Check sheet for the modelled part. Datum: model origin and axes. Units: mm. Face numbers are marked on the shaded views. A direction names the side the tool comes from. Round coordinates to 2 decimals unless told otherwise and drop trailing zeros. Loops run counter-clockwise (first coordinate to the right, second up) from the corner with the lowest first, then second, coordinate; pieces in that order, holes last. Notation, with made-up numbers: (74.25, -30.75) -> (92.25, -30.75) arc R12 ccw to (92.25, -26.75) -> close; hole circle Ø2 at (-13, 23.5). An arc over 180 degrees is marked (long way). Use one line per item in the form item = value. Start each with the question number.
(1) Draft check along Z on the marked faces 1, 2 and 3. Enter one of: released by +Z, released by -Z, zero draft, split by the parting line, or undercut.
(2) Sectioned sample at C-C (y = -15.5). Record the cut outline in (x, z), and give its area (3 significant figures).
(3) Go/stop test with flat-tipped pins: pin 1 (3 mm diameter, centred on x = -6.5, y = 21, fed in from -Z); pin 2 (0.9 mm diameter, centred on x = 9, z = -77.5, fed in from +Y); pin 3 (4 mm diameter, centred on x = 28, y = 9.5, fed in from -Z); pin 4 (0.9 mm diameter, centred on x = -1, z = -77.5, fed in from -Y). Record where each tip stops, or that it passes through.
(4) Set-up check for the marked faces 4 and 5: record each of +Z, -Z, +X, -X, +Y, -Y from which the full face is reachable in a straight line by a thin tool's end or side.
(5) Sectioned sample at B-B (y = 16). Record the cut outline in (x, z).
(6) Sectioned sample at D-D (x = -3). Record the cut outline in (y, z), and give its area (3 significant figures).
(7) Sectioned sample at A-A (z = -43). Record the cut outline in (x, y), and give its area (3 significant figures).
(8) Material ranges on probe 1 along X at (y, z) = (27.8, -43); probe 2 along X at (y, z) = (26, 0); probe 3 along X at (y, z) = (16, -75), recorded low to high. Write a range as [from, to].
from build123d import *

# Parameters (mm, degrees)
SKETCH_1_R               = 5
EXTRUDE_1_DEPTH          = 30
EXTRUDE_1_2_DEPTH        = 30
EXTRUDE_1_3_DEPTH        = 30
EXTRUDE_1_4_DEPTH        = 30
EXTRUDE_START            = 18
SKETCH_2_R               = 5
EXTRUDE_2_DEPTH          = 18
SKETCH_3_R               = 2.1
CUT_EXTRUDE_1_DEPTH      = 5
EXTRUDE_START_2          = 20
EXTRUDE_3_DEPTH          = 10
EXTRUDE_3_2_DEPTH        = 10
CUT_EXTRUDE_2_DEPTH      = 102.257098517
CUT_EXTRUDE_2_DEPTH_BACK = 102.257098517
EXTRUDE_START_3          = -3
EXTRUDE_4_DEPTH          = 3
SKETCH_7_R               = 2.1
CUT_EXTRUDE_3_DEPTH      = 5
SKETCH_8_R               = 1.9
EXTRUDE_5_DEPTH          = 4
SKETCH_9_R               = 1.9
EXTRUDE_6_DEPTH          = 4
CHAMFER_1_SIZE           = 1


with BuildPart() as part:
    # Sketch 1 → Extrude 1 (new body)
    with BuildSketch(Plane(origin=(0, 0, 0), x_dir=(1, 0, 0), z_dir=(0, 1, 0))):
        with Locations(Location((30, 0, 0), (0, 0, 270))):
            Circle(SKETCH_1_R)
    extrude(amount=EXTRUDE_1_DEPTH)



with BuildPart() as body_2:
    # Sketch 1 → Extrude 1 2 (new body)
    with BuildSketch(Plane(origin=(0, 0, 0), x_dir=(1, 0, 0), z_dir=(0, 1, 0))):
        with Locations(Location((25, 77, 0), (0, 0, 270))):
            Circle(SKETCH_1_R)
    extrude(amount=EXTRUDE_1_2_DEPTH)


with BuildPart() as body_3:
    # Sketch 1 → Extrude 1 3 (new body)
    with BuildSketch(Plane(origin=(0, 0, 0), x_dir=(1, 0, 0), z_dir=(0, 1, 0))):
        with Locations(Location((-30, 0, 0), (0, 0, 90))):
            Circle(SKETCH_1_R)
    extrude(amount=EXTRUDE_1_3_DEPTH)


with BuildPart() as body_4:
    # Sketch 1 → Extrude 1 4 (new body)
    with BuildSketch(Plane(origin=(0, 0, 0), x_dir=(1, 0, 0), z_dir=(0, 1, 0))):
        with Locations(Location((-25, 77, 0), (0, 0, 90))):
            Circle(SKETCH_1_R)
    extrude(amount=EXTRUDE_1_4_DEPTH)


with BuildPart() as part_1:
    add(part.part)

    add(body_3.part)  # Extrude 2 merges body 3
    # Sketch 2 → Extrude 2 (add)
    with BuildSketch(Plane.XZ.offset(EXTRUDE_START)):
        with Locations(Location((-30, 0, 0), (0, 0, 270))):
            Circle(SKETCH_2_R)
        with Locations(Location((30, 0, 0), (0, 0, 270))):
            Circle(SKETCH_2_R)
    extrude(amount=-EXTRUDE_2_DEPTH)

    # Sketch 5 → Cut-Extrude 2 (cut, two sides: drawn at the far end of the back side and taken through both)
    with BuildSketch(Plane(origin=(0, 30, 0), x_dir=(1, 0, 0), z_dir=(0, 1, 0)).offset(-CUT_EXTRUDE_2_DEPTH_BACK)):
        with BuildLine():
            Line((-32.175491387, 4.50191484), (-25.273954776, 1.632328565))
            ThreePointArc((-25.273954776, 1.632328565), (-28.080374368, 4.61682114), (-32.175491387, 4.50191484))
        make_face()
        with BuildLine():
            Line((25.273954776, 1.632328565), (32.175491387, 4.50191484))
            ThreePointArc((32.175491387, 4.50191484), (28.080374368, 4.61682114), (25.273954776, 1.632328565))
        make_face()
    extrude(amount=CUT_EXTRUDE_2_DEPTH + CUT_EXTRUDE_2_DEPTH_BACK, mode=Mode.SUBTRACT)



with BuildPart() as cut_extrude_1_tool:
    # Sketch 3 → Cut-Extrude 1 (new body)
    with BuildSketch(Plane(origin=(0, 30, 0), x_dir=(1, 0, 0), z_dir=(0, 1, 0))):
        with Locations(Location((-25, 77, 0), (0, 0, 270))):
            Circle(SKETCH_3_R)
        with Locations(Location((25, 77, 0), (0, 0, 270))):
            Circle(SKETCH_3_R)
    extrude(amount=-CUT_EXTRUDE_1_DEPTH)


with BuildPart() as body_2_1:
    add(body_2.part)

    # Cut-Extrude 1: cut by cut_extrude_1_tool
    add(cut_extrude_1_tool.part, mode=Mode.SUBTRACT)


with BuildPart() as body_4_1:
    add(body_4.part)

    # Cut-Extrude 1: cut by cut_extrude_1_tool
    add(cut_extrude_1_tool.part, mode=Mode.SUBTRACT)


with BuildPart() as body_4_2:
    # Sketch 4 → Extrude 3 (new body)
    with BuildSketch(Plane(origin=(0, 0, 0), x_dir=(1, 0, 0), z_dir=(0, 1, 0)).offset(EXTRUDE_START_2)):
        with BuildLine():
            Line((23, 48), (28.159807037, 48))
            ThreePointArc((28.159807037, 48), (33.159807037, 43), (28.159807037, 38))
            Line((28.159807037, 38), (23, 38))
            Line((23, 38), (23, 48))
        make_face()
    extrude(amount=EXTRUDE_3_DEPTH)


with BuildPart() as body_5:
    # Sketch 4 → Extrude 3 2 (new body)
    with BuildSketch(Plane(origin=(0, 0, 0), x_dir=(1, 0, 0), z_dir=(0, 1, 0)).offset(EXTRUDE_START_2)):
        with BuildLine():
            Line((-23, 48), (-28.159807037, 48))
            ThreePointArc((-28.159807037, 48), (-33.159807037, 43), (-28.159807037, 38))
            Line((-28.159807037, 38), (-23, 38))
            Line((-23, 38), (-23, 48))
        make_face()
    extrude(amount=EXTRUDE_3_2_DEPTH)


with BuildPart() as part_2:
    add(part_1.part)

    add(body_2_1.part)  # Extrude 4 merges body 2

    add(body_4_1.part)  # Extrude 4 merges body 4

    add(body_4_2.part)  # Extrude 4 merges body 4 2

    add(body_5.part)  # Extrude 4 merges body 5
    # Sketch 6 → Extrude 4 (add)
    with BuildSketch(Plane(origin=(0, 30, 0), x_dir=(1, 0, 0), z_dir=(0, 1, 0)).offset(EXTRUDE_START_3)):
        Polygon((-29.42411231, 1.385046342), (-38.5, 5.158704907), (-38.5, 28.603878074), (-26.710319101, 42.386930811), (-23.632939423, 75.5), (23.632939423, 75.5), (26.710319101, 42.386930811), (38.5, 28.603878074), (38.5, 5.158704907), (29.42411231, 1.385046342), (30.57588769, -1.385046342), (41.5, 3.157084566), (41.5, 29.7119114), (29.609294973, 43.613069189), (26.367060577, 78.5), (-26.367060577, 78.5), (-29.609294973, 43.613069189), (-41.5, 29.7119114), (-41.5, 3.157084566), (-30.57588769, -1.385046342), align=None)
    extrude(amount=-EXTRUDE_4_DEPTH)

    # Sketch 7 → Cut-Extrude 3 (cut)
    with BuildSketch(Plane(origin=(0, 30, 0), x_dir=(1, 0, 0), z_dir=(0, 1, 0))):
        with Locations(Location((30, 0, 0), (0, 0, 270))):
            Circle(SKETCH_7_R)
        with Locations(Location((-30, 0, 0), (0, 0, 270))):
            Circle(SKETCH_7_R)
        with Locations(Location((28.159807037, 43, 0), (0, 0, 270))):
            Circle(SKETCH_7_R)
        with Locations(Location((-28.159807037, 43, 0), (0, 0, 270))):
            Circle(SKETCH_7_R)
        with Locations(Location((25, 77, 0), (0, 0, 270))):
            Circle(SKETCH_7_R)
        with Locations(Location((-25, 77, 0), (0, 0, 270))):
            Circle(SKETCH_7_R)
    extrude(amount=-CUT_EXTRUDE_3_DEPTH, mode=Mode.SUBTRACT)

    # Sketch 8 → Extrude 5 (add)
    with BuildSketch(Plane.XZ.offset(18)):
        with Locations(Location((-30, 0, 0), (0, 0, 270))):
            Circle(SKETCH_8_R)
        with Locations(Location((30, 0, 0), (0, 0, 270))):
            Circle(SKETCH_8_R)
    extrude(amount=EXTRUDE_5_DEPTH)

    # Sketch 9 → Extrude 6 (add)
    with BuildSketch(Plane.XZ):
        with Locations(Location((-25, -77, 0), (0, 0, 270))):
            Circle(SKETCH_9_R)
        with Locations(Location((25, -77, 0), (0, 0, 270))):
            Circle(SKETCH_9_R)
    extrude(amount=EXTRUDE_6_DEPTH)

    # Chamfer 1
    chamfer_1_edges = [part_2.edges().sort_by_distance(p)[0] for p in [
        (-28.159807037, 30, -45.1),
        (28.159807037, 30, -45.1),
        (-30, 30, -2.1),
        (30, 30, -2.1),
        (-30, -22, 1.9),
        (30, -22, 1.9),
        (-25, -4, -75.1),
        (25, -4, -75.1),
        (-25, 30, -79.1),
        (25, 30, -79.1),
    ]]
    chamfer(chamfer_1_edges, length=CHAMFER_1_SIZE)


solid = part_2.part
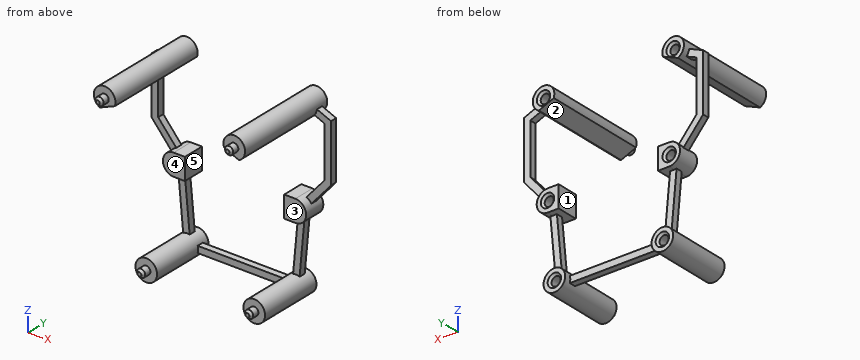
Checks:
q1.face_1 = zero draft
q1.face_2 = undercut
q1.face_3 = undercut
q2.outline = (-32.18, -4.5) -> (-25.27, -1.63) arc R5 ccw (long way) to start; (25.27, -1.63) -> (32.18, -4.5) arc R5 ccw (long way) to start
q2.area = 140 mm2
q3.pin_1 = through
q3.pin_2 = 27
q3.pin_3 = -81.9
q3.pin_4 = 24
q4.face_4 = +X, -X, -Y
q4.face_5 = +Z, +Y, -Y
q5.outline = (-32.18, -4.5) -> (-25.27, -1.63) arc R5 ccw (long way) to start; circle Ø10 at (-25, -77); circle Ø10 at (25, -77); (25.27, -1.63) -> (32.18, -4.5) arc R5 ccw (long way) to start
q6.outline = (24, -78.5) -> (27, -78.5) -> (27, -75.5) -> (24, -75.5) -> close
q6.area = 9.00 mm2
q7.outline = (-33.16, 20) -> (-23, 20) -> (-23, 30) -> (-25.06, 30) -> (-26.06, 29) -> (-26.06, 25) -> (-30.26, 25) -> (-30.26, 29) -> (-31.26, 30) -> (-33.16, 30) -> close; (23, 20) -> (33.16, 20) -> (33.16, 30) -> (31.26, 30) -> (30.26, 29) -> (30.26, 25) -> (26.06, 25) -> (26.06, 29) -> (25.06, 30) -> (23, 30) -> close
q7.area = 159 mm2
q8.probe_1 = [-33.16, -30.26], [-26.06, -23], [23, 26.06], [30.26, 33.16]
q8.probe_2 = [-35, -32.1], [-27.9, -25], [25, 27.9], [32.1, 35]
q8.probe_3 = [-29.58, -20.42], [20.42, 29.58]
